```python
from build123d import *

# Parameters (mm, degrees)
SKETCH1_W        = 20
SKETCH1_H        = 26
BASE_DEPTH       = 1.5
SKETCH3_W        = 1.5
SKETCH3_H        = 6
MOUNT_EARS_DEPTH = 1.5
RIBS_REACH       = 47.875


with BuildPart() as part:
    # Sketch1 → Base (new body)
    with BuildSketch(Plane.XY):
        with Locations((10, 27.497191913)):
            Rectangle(SKETCH1_W, SKETCH1_H)
    extrude(amount=BASE_DEPTH)

    # Sketch3 → Mount ears (add)
    with BuildSketch(Plane.XY.offset(1.5)):
        with Locations((-0.75, 33.997191913)):
            Rectangle(SKETCH3_W, SKETCH3_H)
        with Locations((20.75, 33.997191913)):
            Rectangle(SKETCH3_W, SKETCH3_H)
        with Locations((20.75, 20.997191913)):
            Rectangle(SKETCH3_W, SKETCH3_H)
        with Locations((-0.75, 20.997191913)):
            Rectangle(SKETCH3_W, SKETCH3_H)
    extrude(amount=-MOUNT_EARS_DEPTH)

    # Sketch5 → Ribs (cut, up to next)
    with BuildSketch(Plane.XY.offset(1.5), mode=Mode.PRIVATE) as ribs_sk1:
        with BuildLine():
            Line((4, 37.497191913), (16, 37.497191913))
            ThreePointArc((16, 37.497191913), (17, 36.497191913), (16, 35.497191913))
            Line((16, 35.497191913), (4, 35.497191913))
            ThreePointArc((4, 35.497191913), (3, 36.497191913), (4, 37.497191913))
        make_face()
    ribs_tool1 = extrude(ribs_sk1.sketch, amount=-RIBS_REACH, mode=Mode.PRIVATE) & part.part
    # Sketch5 → Ribs (cut, up to next)
    with BuildSketch(Plane.XY.offset(1.5), mode=Mode.PRIVATE) as ribs_sk2:
        with BuildLine():
            Line((4, 32.997191913), (16, 32.997191913))
            ThreePointArc((16, 32.997191913), (17, 31.997191913), (16, 30.997191913))
            Line((16, 30.997191913), (4, 30.997191913))
            ThreePointArc((4, 30.997191913), (3, 31.997191913), (4, 32.997191913))
        make_face()
    ribs_tool2 = extrude(ribs_sk2.sketch, amount=-RIBS_REACH, mode=Mode.PRIVATE) & part.part
    # Sketch5 → Ribs (cut, up to next)
    with BuildSketch(Plane.XY.offset(1.5), mode=Mode.PRIVATE) as ribs_sk3:
        with BuildLine():
            Line((4, 28.497191913), (16, 28.497191913))
            ThreePointArc((16, 28.497191913), (17, 27.497191913), (16, 26.497191913))
            Line((16, 26.497191913), (4, 26.497191913))
            ThreePointArc((4, 26.497191913), (3, 27.497191913), (4, 28.497191913))
        make_face()
    ribs_tool3 = extrude(ribs_sk3.sketch, amount=-RIBS_REACH, mode=Mode.PRIVATE) & part.part
    # Sketch5 → Ribs (cut, up to next)
    with BuildSketch(Plane.XY.offset(1.5), mode=Mode.PRIVATE) as ribs_sk4:
        with BuildLine():
            Line((4, 23.997191913), (16, 23.997191913))
            ThreePointArc((16, 23.997191913), (17, 22.997191913), (16, 21.997191913))
            Line((16, 21.997191913), (4, 21.997191913))
            ThreePointArc((4, 21.997191913), (3, 22.997191913), (4, 23.997191913))
        make_face()
    ribs_tool4 = extrude(ribs_sk4.sketch, amount=-RIBS_REACH, mode=Mode.PRIVATE) & part.part
    # Sketch5 → Ribs (cut, up to next)
    with BuildSketch(Plane.XY.offset(1.5), mode=Mode.PRIVATE) as ribs_sk5:
        with BuildLine():
            Line((4, 19.497191913), (16, 19.497191913))
            ThreePointArc((16, 19.497191913), (17, 18.497191913), (16, 17.497191913))
            Line((16, 17.497191913), (4, 17.497191913))
            ThreePointArc((4, 17.497191913), (3, 18.497191913), (4, 19.497191913))
        make_face()
    ribs_tool5 = extrude(ribs_sk5.sketch, amount=-RIBS_REACH, mode=Mode.PRIVATE) & part.part
    add(ribs_tool1.solids().sort_by_distance((10, 36.497192, 1.5))[0], mode=Mode.SUBTRACT)
    add(ribs_tool2.solids().sort_by_distance((10, 31.997192, 1.5))[0], mode=Mode.SUBTRACT)
    add(ribs_tool3.solids().sort_by_distance((10, 27.497192, 1.5))[0], mode=Mode.SUBTRACT)
    add(ribs_tool4.solids().sort_by_distance((10, 22.997192, 1.5))[0], mode=Mode.SUBTRACT)
    add(ribs_tool5.solids().sort_by_distance((10, 18.497192, 1.5))[0], mode=Mode.SUBTRACT)


solid = part.part
```
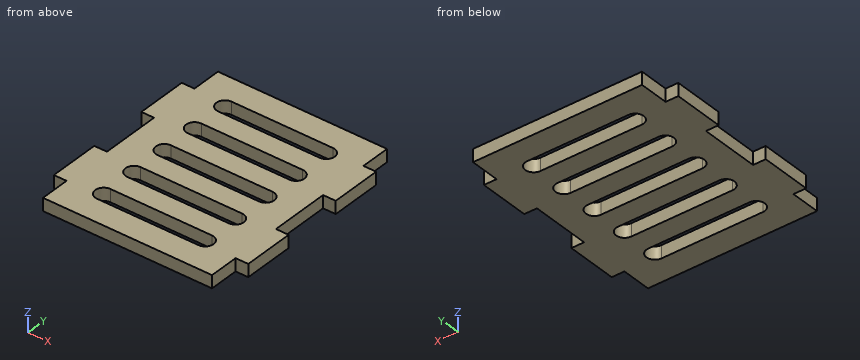
Geometry: final body of the model. Coordinates: model frame, mm. Round coordinates to 2 decimals unless told otherwise and drop trailing zeros. Order: outer loops, then holes, each group sorted by start corner. A loop starts at its lowest first (then second) coordinate and runs counter-clockwise, first axis right, second up. Notation, with made-up numbers: (55, 44) -> (91, 44) arc R31 cw to (91, 69) -> close; hole circle Ø4 at (39.5, -8). An arc over 180 degrees is marked (long way). Write each question's results on one line, items separated by ' | '.
Q1. Section query A-A (x = 5). Output: boundary loops of the cut face in (y, z), and give its area (3 significant figures).
Response values:
outline: (14.5, 0) -> (17.5, 0) -> (17.5, 1.5) -> (14.5, 1.5) -> close; (19.5, 0) -> (22, 0) -> (22, 1.5) -> (19.5, 1.5) -> close; (24, 0) -> (26.5, 0) -> (26.5, 1.5) -> (24, 1.5) -> close; (28.5, 0) -> (31, 0) -> (31, 1.5) -> (28.5, 1.5) -> close; (33, 0) -> (35.5, 0) -> (35.5, 1.5) -> (33, 1.5) -> close; (37.5, 0) -> (40.5, 0) -> (40.5, 1.5) -> (37.5, 1.5) -> close | area: 24.0 mm²
Q2. Section query C-C (z = 0.85). Count the separate pieces of the cut face and the enclosed holes in it, and give its area (3 significant figures).
Response values:
separate pieces: 1 | enclosed holes: 5 | area: 420 mm²
Q3. Ray query, line 1 along Y through (x, z) = (12.25, 0.25); line 2 along Y through (x, z) = (16.5, 1.1); line 3 along X through (y, z) = (30.25, 1.4). Return the intervals inside material, ascending.
Response values:
line 1: 14.5 to 17.5, 19.5 to 22, 24 to 26.5, 28.5 to 31, 33 to 35.5, 37.5 to 40.5 | line 2: 14.5 to 17.63, 19.36 to 22.13, 23.86 to 26.63, 28.36 to 31.13, 32.86 to 35.63, 37.36 to 40.5 | line 3: 0 to 20
Q4. Section query B-B (y = 27.25). Output: boundary loops of the cut face in (x, z), and give its area (3 significant figures).
Response values:
outline: (0, 0) -> (3.03, 0) -> (3.03, 1.5) -> (0, 1.5) -> close; (16.97, 0) -> (20, 0) -> (20, 1.5) -> (16.97, 1.5) -> close | area: 9.09 mm²
Q5. Pin query (flat end, axial travel): pin 1 Ø0.8 at (y, z) = (15.5, 0.5) entering from +X; pin 2 Ø0.8 at (x, z) = (-0.5, 1) entering from -Y; pin 3 Ø0.8 at (x, z) = (-1, 0.5) entering from +Y. Return the tip coordinate at first contact, or that it passes through.
Response values:
pin 1: x = 20 | pin 2: y = 18 | pin 3: y = 37
